from build123d import *

# Parameters (mm, degrees)
PAD_DEPTH           = 7.4
SKETCH095_W         = 4
SKETCH095_H         = 5.5
POCKET045_DEPTH     = 6
PAD048_DEPTH        = 7.4
LINEARPATTERN_COUNT = 6
LINEARPATTERN_PITCH = 1.133333
FILLET_R            = 0.2
FILLET034_R         = 1
CHAMFER028_SIZE     = 0.3
CHAMFER029_SIZE     = 1


with BuildPart() as part:
    # Sketch → Pad (new body)
    with BuildSketch(Plane.XZ):
        Polygon((-6.5, 0), (6.5, 0), (6.5, 2.8), (3.4, 2.8), (3.4, 9.5), (-3.4, 9.5), (-3.4, 2.8), (-6.5, 2.8), align=None)
    extrude(amount=PAD_DEPTH)

    # Sketch095 → Pocket045 (cut)
    with BuildSketch(Plane.XZ):
        with Locations((0, 2.75)):
            Rectangle(SKETCH095_W, SKETCH095_H)
    extrude(amount=POCKET045_DEPTH, mode=Mode.SUBTRACT)

    # Sketch096 → Pad048 (join)
    with BuildSketch(Plane.XZ):
        Polygon((-3.4, 9.5), (-2.266667, 9.5), (-2.833333, 10.481495), align=None)
    pad048 = extrude(amount=PAD048_DEPTH)

    # LinearPattern: Pad048 ×6
    with Locations(*[(i * LINEARPATTERN_PITCH, 0, 0) for i in range(1, LINEARPATTERN_COUNT)]):
        add(pad048)

    # Fillet
    fillet_edges = [part.edges().sort_by_distance(p)[0] for p in [
        (-2.833333, -3.7, 10.481495),
        (-1.7, -3.7, 10.481495),
        (-0.566667, -3.7, 10.481495),
        (0.566667, -3.7, 10.481495),
        (1.7, -3.7, 10.481495),
        (2.833334, -3.7, 10.481495),
    ]]
    fillet(fillet_edges, radius=FILLET_R)

    # Fillet034
    fillet034_edges = [part.edges().sort_by_distance(p)[0] for p in [
        (-6.5, 0, 1.4),
        (-6.5, -7.4, 1.4),
        (6.5, -7.4, 1.4),
        (6.5, 0, 1.4),
    ]]
    fillet(fillet034_edges, radius=FILLET034_R)

    # Chamfer028
    chamfer028_edges = [part.edges().sort_by_distance(p)[0] for p in [
        (-3.75, 0, 0),
        (-6.207107, -0.292893, 0),
        (-2, -3, 0),
        (-6.5, -3.7, 0),
        (0, -6, 0),
        (-6.207107, -7.107107, 0),
        (2, -3, 0),
        (0, -7.4, 0),
        (3.75, 0, 0),
        (6.207107, -7.107107, 0),
        (6.207107, -0.292893, 0),
        (6.5, -3.7, 0),
    ]]
    chamfer(chamfer028_edges, length=CHAMFER028_SIZE)

    # Chamfer029
    chamfer029_edges = [part.edges().sort_by_distance(p)[0] for p in [
        (2, -3, 5.5),
        (-2, -3, 5.5),
    ]]
    chamfer(chamfer029_edges, length=CHAMFER029_SIZE)


with BuildPart() as part_1:
    # Body placement: moved
    add(part.part.moved(Location((-5, 14.5, 7.2))))


solid = part_1.part
Could you check a few things on this model? Use its own coordinates, in mm. A direction names the side the tool comes from. Coordinates: 2 decimals unless noted, no trailing zeros. Loops run counter-clockwise (first coordinate to the right, second up) from the corner with the lowest first, then second, coordinate; pieces in that order, holes last. Notation, with made-up numbers: (-26, 18) -> (10, 18) arc R13 cw to (10, 28) -> close; hole circle Ø3 at (-18, -8.5). An arc over 180 degrees is marked (long way). Answer in a Markdown table with one row per item.
(1) Imagine slicing it at C-C (z = 11.5). List the corners of the cut face in (x, y) for me.
Results found:
| item | result |
|---|---|
| outline | (-8.4, 7.1) -> (-1.6, 7.1) -> (-1.6, 14.5) -> (-3, 14.5) -> (-3, 8.5) -> (-7, 8.5) -> (-7, 14.5) -> (-8.4, 14.5) -> close |
(2) Imagine slicing it at D-D (x = -2.5). List the corners of the cut face in (y, z) for me.
Results found:
| item | result |
|---|---|
| outline | (7.1, 7.5) -> (7.4, 7.2) -> (14.2, 7.2) -> (14.5, 7.5) -> (14.5, 17.1) -> (7.1, 17.1) -> close |
(3) If I drill on probe 1 along X at (y, z) = (8.75, 11); probe 2 along X at (y, z) = (9.5, 9.75); probe 3 along X at (y, z) = (10.5, 17.25), over which ranges is the centre line in solid material (lowest first)?
Results found:
| item | result |
|---|---|
| probe 1 | x = -8.4 to -7, -3 to -1.6 |
| probe 2 | x = -11.5 to -7, -3 to 1.5 |
| probe 3 | x = -8.08 to -7.58, -6.95 to -6.45, -5.82 to -5.32, -4.68 to -4.18, -3.55 to -3.05, -2.42 to -1.92 |
(4) For faces 4 (the face through (-11.199, 7.385, 8.732)), 5 (the face through (-5, 12, 12.7)), 6 (the face through (-10, 11, 10)), 7 (the face through (-1.6, 11, 13)), which set-ups out of +Z, -Z, +X, -X, +Y, -Y let a thin tool reach every point of the face, with its end or its side?
Results found:
| item | result |
|---|---|
| face 4 | +Z, -Z, -X, -Y |
| face 5 | -Z, +Y |
| face 6 | +Z, -X, +Y, -Y |
| face 7 | +Z, +X, +Y, -Y |
(5) Imagine slicing it at A-A (z = 9.75). List the corners of the cut face in (x, y) for me, plus the area to 3 significant figures.
Results found:
| item | result |
|---|---|
| outline | (-11.5, 8.1) arc R1 ccw to (-10.5, 7.1) -> (0.5, 7.1) arc R1 ccw to (1.5, 8.1) -> (1.5, 13.5) arc R1 ccw to (0.5, 14.5) -> (-3, 14.5) -> (-3, 8.5) -> (-7, 8.5) -> (-7, 14.5) -> (-10.5, 14.5) arc R1 ccw to (-11.5, 13.5) -> close |
| area | 71.3 mm^2 |
(6) Will these pins go through, and if not, where does the flat tip stop? pin 1 Ø3 at (x, z) = (-5, 9.5) entering from +Y; pin 2 Ø1.6 at (x, y) = (-5, 10) entering from -Z; pin 3 Ø3.5 at (y, z) = (11, 14.5) entering from -X.
Results found:
| item | result |
|---|---|
| pin 1 | stops at y = 8.5 |
| pin 2 | stops at z = 12.7 |
| pin 3 | stops at x = -8.4 |
(7) Imagine slicing it at B-B (x = -9.5). List the corners of the cut face in (y, z) for me, plus the area to 3 significant figures.
Results found:
| item | result |
|---|---|
| outline | (7.1, 7.5) -> (7.4, 7.2) -> (14.2, 7.2) -> (14.5, 7.5) -> (14.5, 10) -> (7.1, 10) -> close |
| area | 20.6 mm^2 |
(8) Thinking about a two-plate mould opening in X: for faces 1 (the face through (-6.5, 11.5, 12.2)), 2 (the face through (-8.4, 11, 13)), 3 (the face through (1.199, 7.385, 8.768)), which applies, released by +X, released by -X, zero draft, split by the parting line, or undercut?
Results found:
| item | result |
|---|---|
| face 1 | undercut |
| face 2 | released by -X |
| face 3 | released by +X |
